Input: part model. Units: mm. Frame: model coordinates. Face numbers are marked on the shaded views. A direction names the side the tool comes from. Give positions to 0.01 mm unless a question says otherwise; leave off trailing zeros. Loops run counter-clockwise (first coordinate to the right, second up) from the corner with the lowest first, then second, coordinate; pieces in that order, holes last.
Autodesk Inventor part; units mm, degrees
ref_plane "Work Plane1" through (0, -44, 0) normal (0, -1, 0) x (1, 0, 0)
ref_plane "Work Plane2" through (0, 40, 0) normal (0, 1, 0) x (1, 0, 0)
ref_plane "Work Plane3" through (0, 50, 0) normal (0, 1, 0) x (1, 0, 0)
sketch "Sketch1" plane through (0, 0, 0) normal (0, 1, 0) x (-1, 0, 0)
  circle A0 centre (0, 0) radius 16.5
  dimension "d0" = 33
extrude "Extrusion1" add sketch "Sketch1" along normal blind 25
ref_plane "Work Plane1" through (0, -44, 0) normal (0, -1, 0) x (1, 0, 0)
sketch "Sketch2" plane through (0, -44, 0) normal (0, -1, 0) x (1, 0, 0)
  circle A0 centre (0, 0) radius 15
  dimension "d4" = 30
loft "Loft1" add profiles "Sketch2" section 1 edges at (16.5, 0, 0)
ref_plane "Work Plane2" through (0, 40, 0) normal (0, 1, 0) x (1, 0, 0)
sketch "Sketch3" plane through (0, 40, 0) normal (0, 1, 0) x (1, 0, 0)
  circle A0 centre (0, 0) radius 15
  dimension "d10" = 30
loft "Loft2" add profiles "Sketch3" section 1 edges at (16.5, 25, 0)
ref_plane "Work Plane3" through (0, 50, 0) normal (0, 1, 0) x (1, 0, 0)
sketch "Sketch4" plane through (0, 50, 0) normal (0, 1, 0) x (1, 0, 0)
  circle A0 centre (0, 0) radius 10
  dimension "d16" = 20
loft "Loft3" add profiles "Sketch4" section 1 edges at (15, 40, 0)
properties part number "USBCamera"
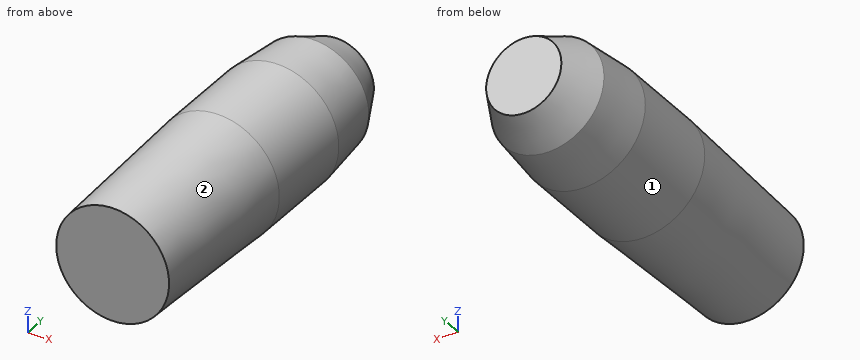
(1) Cut plane C-C (y = 37). Return the cut outline in (x, z).
Values follow:
outline: circle Ø30.6 at (0, 0)
(2) Reachability of the marked faces 1 and 2 from +Z, -Z, +X, -X, +Y, -Y: full face, straight path, thin tool, end or side. Return the list, or none.
Values follow:
face 1: +Y, -Y
face 2: -Y
(3) Cut plane B-B (y = 5.5). Return the cut outline in (x, z).
Values follow:
outline: circle Ø33 at (0, 0)
(4) Ray query, probe 1 along X at (y, z) = (20, -12.5); probe 2 along X at (y, z) = (36, -5); probe 3 along Y at (x, z) = (4.5, 13). Return the intervals inside material, ascending.
Values follow:
probe 1: x = -10.77 to 10.77
probe 2: x = -14.57 to 14.57
probe 3: y = -44 to 42.49
(5) Cut plane A-A (x = 0). Return the cut outline in (y, z).
Values follow:
outline: (-44, -15) - (0, -16.5) - (25, -16.5) - (40, -15) - (50, -10) - (50, 10) - (40, 15) - (25, 16.5) - (0, 16.5) - (-44, 15) - close
(6) Pin query (flat end, axial travel): pin 1 Ø8 at (y, z) = (14.5, 10.5) entering from +X; pin 2 Ø1 at (x, y) = (5, -21) entering from +Z; pin 3 Ø10 at (x, y) = (12.5, -18.5) entering from -Z; pin 4 Ø10 at (x, y) = (3.5, -3) entering from +Z. Return the tip coordinate at first contact, or that it passes through.
Values follow:
pin 1: stops at x = 15.17
pin 2: stops at z = 15.13
pin 3: stops at z = -13.99
pin 4: stops at z = 16.5
